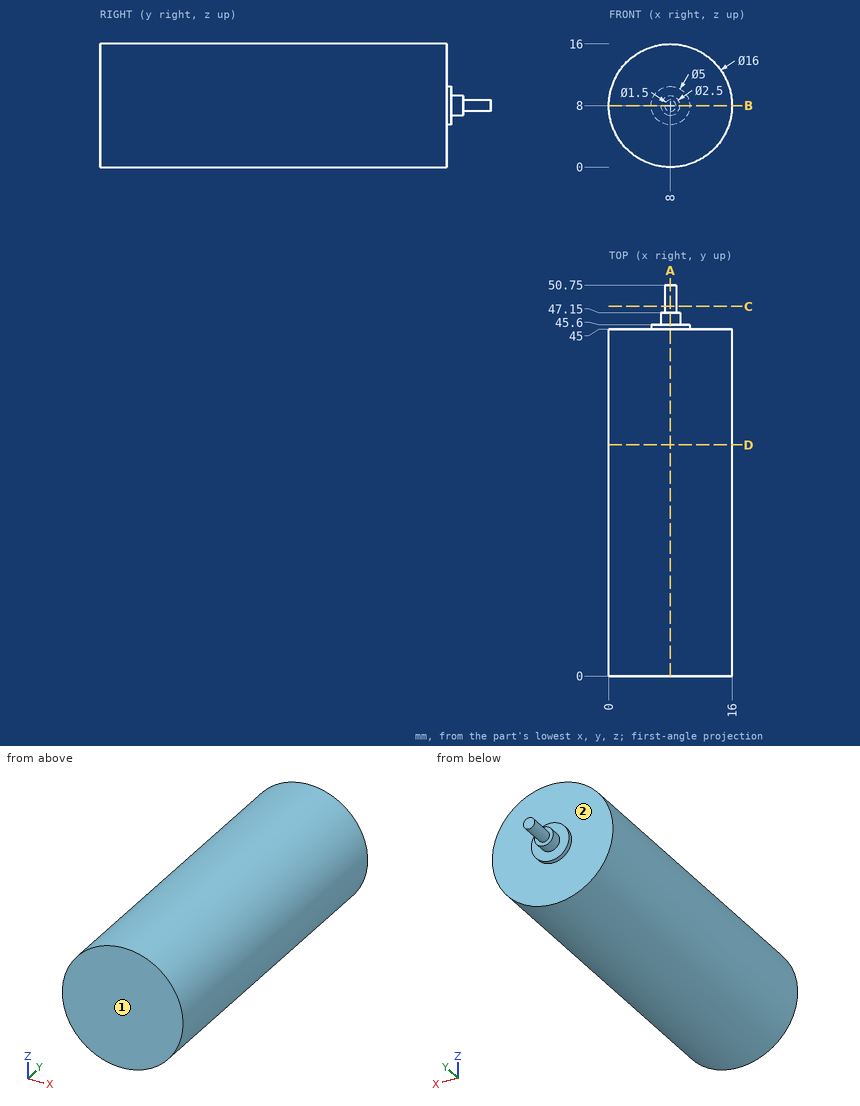
The figure shows three views and two pictorial views of one solid part (mm, origin at its lowest corner). Answer the questions. A direction names the side the tool comes from. Coordinates: 2 decimals unless noted, no trailing zeros. Loops run counter-clockwise (first coordinate to the right, second up) from the corner with the lowest first, then second, coordinate; pieces in that order, holes last.
1) Find section D-D on y = 30. Write down the section's boundary in (x, z).
2) Find section A-A on x = 8. Write down the section's boundary in (y, z), then the cut area to 3 significant figures.
3) Find the intervals of material crossed by L1, parallel to Y at x = 4.5, z = 15; L2, parallel to Z at x = 1, y = 24; L3, parallel to Z at x = 4, y = 36, in increasing order.
4) A tool of negligible diameter and unlimited length cuts with its end or side. For the marked faces 1 and 2, from which of +Z, -Z, +X, -X, +Y, -Y can it reach the whole face along a straight path? Write none if from no direction.
5) Flat-ended cylindrical pins translate along their axes: pin 1 Ø1 at (y, z) = (8, 7) entering from +X; pin 2 Ø3 at (x, y) = (13.5, 42.5) entering from -Z; pin 3 Ø3 at (x, z) = (5.5, 2) entering from +Y. Find the tip coordinate at first contact, or state that the pin passes through.
6) Find section C-C on y = 48. Write down the section's boundary in (x, z).
7) Find section B-B on z = 8. Write down the section's boundary in (x, y), then the cut area to 3 significant figures.
Values:
1. outline: circle Ø16 at (8, 8)
2. outline: (0, 0) - (45, 0) - (45, 5.5) - (45.6, 5.5) - (45.6, 6.75) - (47.15, 6.75) - (47.15, 7.25) - (50.75, 7.25) - (50.75, 8.75) - (47.15, 8.75) - (47.15, 9.25) - (45.6, 9.25) - (45.6, 10.5) - (45, 10.5) - (45, 16) - (0, 16) - close
2. area: 732 mm2
3. L1: y = 0 to 45
3. L2: z = 4.13 to 11.87
3. L3: z = 1.07 to 14.93
4. face 1: +Z, -Z, +X, -X, -Y
4. face 2: +Y
5. pin 1: stops at x = 15.98
5. pin 2: stops at z = 1.07
5. pin 3: stops at y = 45
6. outline: circle Ø1.5 at (8, 8)
7. outline: (0, 0) - (16, 0) - (16, 45) - (10.5, 45) - (10.5, 45.6) - (9.25, 45.6) - (9.25, 47.15) - (8.75, 47.15) - (8.75, 50.75) - (7.25, 50.75) - (7.25, 47.15) - (6.75, 47.15) - (6.75, 45.6) - (5.5, 45.6) - (5.5, 45) - (0, 45) - close
7. area: 732 mm2
